Work out the finished part from the listing and answer in its coordinate system (mm). A direction names the side the tool comes from. Round coordinates to 2 decimals unless told otherwise and drop trailing zeros. Order: outer loops, then holes, each group sorted by start corner. A loop starts at its lowest first (then second) coordinate and runs counter-clockwise, first axis right, second up.
from build123d import *

# Parameters (mm, degrees)
SKETCH1_W           = 120
SKETCH1_H           = 25
SKETCH1_R           = 1.5
BOSS_EXTRUDE1_DEPTH = 4
SKETCH2_W           = 7
SKETCH2_H           = 4
BOSS_EXTRUDE2_DEPTH = 8


with BuildPart() as part:
    # Sketch1 → Boss-Extrude1 (new body)
    with BuildSketch(Plane(origin=(0, 0, 0), x_dir=(1, 0, 0), z_dir=(0, 1, 0))):
        Rectangle(SKETCH1_W, SKETCH1_H)
        with Locations(Location((40, 5, 0), (0, 0, 270))):
            Circle(SKETCH1_R, mode=Mode.SUBTRACT)
        with Locations(Location((40, -5, 0), (0, 0, 90))):
            Circle(SKETCH1_R, mode=Mode.SUBTRACT)
        with Locations(Location((50, 5, 0), (0, 0, 270))):
            Circle(SKETCH1_R, mode=Mode.SUBTRACT)
        with Locations(Location((50, -5, 0), (0, 0, 90))):
            Circle(SKETCH1_R, mode=Mode.SUBTRACT)
        with BuildLine():
            ThreePointArc((31.321653543, 0.599330025), (31.95, 0), (31.321653543, -0.599330025))
            ThreePointArc((31.321653543, -0.599330025), (18.65, 0), (31.321653543, 0.599330025))
        make_face(mode=Mode.SUBTRACT)
        with BuildLine():
            ThreePointArc((6.321653543, 0.599330025), (6.95, 0), (6.321653543, -0.599330025))
            ThreePointArc((6.321653543, -0.599330025), (-6.35, 0), (6.321653543, 0.599330025))
        make_face(mode=Mode.SUBTRACT)
        with BuildLine():
            ThreePointArc((-18.678346457, 0.599330025), (-18.05, 0), (-18.678346457, -0.599330025))
            ThreePointArc((-18.678346457, -0.599330025), (-31.35, 0), (-18.678346457, 0.599330025))
        make_face(mode=Mode.SUBTRACT)
    extrude(amount=BOSS_EXTRUDE1_DEPTH)

    # Sketch2 → Boss-Extrude2 (add)
    with BuildSketch(Plane.ZY.offset(60)):
        with Locations((-9, 2)):
            Rectangle(SKETCH2_W, SKETCH2_H)
        with Locations((9, 2)):
            Rectangle(SKETCH2_W, SKETCH2_H)
    boss_extrude2 = extrude(amount=BOSS_EXTRUDE2_DEPTH)

    # Mirror1: Boss-Extrude2 across plane
    add(boss_extrude2.mirror(Plane.ZY))


solid = part.part
Item 1: For a pull along X with two mould halves and no side action, classify faces 1 (the face through (-64, 2, 5.5)), 2 (the face through (-60, 2, 0)), 3 (the face through (51.464, 1.972, 5.325)) as released by +X, released by -X, zero draft, split by the parting line, or undercut.
Item 2: A tool of negligible diameter and unlimited length cuts with its end or side. For faces 4 (the face through (64, 2, -5.5)), 5 (the face through (18.656, 1.972, 0.271)), 6 (the face through (-64, 2, -5.5)), from which of +Z, -Z, +X, -X, +Y, -Y can it reach the whole face along a straight path? Write none if from no direction.
Item 3: Find section C-C (z = -1.75). Write down the section's boundary in (x, y), plus the area to 3 significant figures.
Item 4: Find section A-A (x = 50). Write down the section's boundary in (y, z), plus the area to 3 significant figures.
Item 5: Find section B-B (x = -25). Write down the section's boundary in (y, z).
Item 6: Find section D-D (y = 3.15). Write down the section's boundary in (x, z).
Item 7: Given pin 1 (2 mm diameter, centred on y = 2, z = 2, fed in from +X); pin 2 (1.2 mm diameter, centred on y = 1.5, z = -1, fed in from -X), each flat-ended and moving along its own axis, determine where each tip first touches the part or whether it passes through.
Item 8: Find the intervals of material crossed by line 1 along X through (y, z) = (1.25, -5); line 2 along X through (y, z) = (3.4, -2); line 3 along Z through (x, y) = (0, 0.95), in increasing order.
Model answer:
1. face 1: zero draft
1. face 2: released by -X
1. face 3: undercut
2. face 4: +X, +Y, -Y
2. face 5: +Y, -Y
2. face 6: -X, +Y, -Y
3. outline: (-60, 0) - (-31.1, 0) - (-31.1, 4) - (-60, 4) - close; (-18.9, 0) - (-6.1, 0) - (-6.1, 4) - (-18.9, 4) - close; (6.1, 0) - (18.9, 0) - (18.9, 4) - (6.1, 4) - close; (31.1, 0) - (60, 0) - (60, 4) - (31.1, 4) - close
3. area: 334 mm2
4. outline: (0, -12.5) - (4, -12.5) - (4, -6.5) - (0, -6.5) - close; (0, -3.5) - (4, -3.5) - (4, 3.5) - (0, 3.5) - close; (0, 6.5) - (4, 6.5) - (4, 12.5) - (0, 12.5) - close
4. area: 76.0 mm2
5. outline: (0, -12.5) - (4, -12.5) - (4, -6.35) - (0, -6.35) - close; (0, 6.35) - (4, 6.35) - (4, 12.5) - (0, 12.5) - close
6. outline: (-68, -12.5) - (68, -12.5) - (68, -5.5) - (60, -5.5) - (60, 5.5) - (68, 5.5) - (68, 12.5) - (-68, 12.5) - (-68, 5.5) - (-60, 5.5) - (-60, -5.5) - (-68, -5.5) - close; hole (-18.68, -0.6) arc R0.6 ccw (long way) to (-18.68, 0.6) arc R6.35 ccw (long way) to start; hole (6.32, -0.6) arc R0.6 ccw (long way) to (6.32, 0.6) arc R6.35 ccw (long way) to start; hole (31.32, -0.6) arc R0.6 ccw (long way) to (31.32, 0.6) arc R6.35 ccw (long way) to start; hole circle Ø3 at (40, -5); hole circle Ø3 at (40, 5); hole circle Ø3 at (50, -5); hole circle Ø3 at (50, 5)
7. pin 1: stops at x = 60
7. pin 2: stops at x = -60
8. line 1: x = -60 to -28.91, -21.09 to -3.91, 3.91 to 21.09, 28.91 to 38.5, 41.5 to 48.5, 51.5 to 60
8. line 2: x = -60 to -31.03, -18.97 to -6.03, 6.03 to 18.97, 31.03 to 60
8. line 3: z = -12.5 to -6.35, 6.35 to 12.5
